Check sheet for the modelled part. Datum: model origin and axes. Units: mm. A direction names the side the tool comes from. Round coordinates to 2 decimals unless told otherwise and drop trailing zeros. Order: outer loops, then holes, each group sorted by start corner. A loop starts at its lowest first (then second) coordinate and runs counter-clockwise, first axis right, second up.
(1) Sectioned sample at A-A, the plane z = 15. Enter the section's corners in (x, y).
(2) Tool access check on faces 4 (the flat face through (0, -10, 28)), 5 (the flat face through (-15, 3, 0)), 6 (the flat face through (15, 3, 0)). Record the directions out of +Z, -Z, +X, -X, +Y, -Y that give a thin tool (end or side, any length) a straight path to the whole face; none if there is none.
(3) Depth check by flat-ended pin: pin 1 (4 mm diameter, centred on x = -6.5, z = -15, fed in from +Y); pin 2 (5 mm diameter, centred on x = 15, z = -8, fed in from -Y); pin 3 (6.5 mm diameter, centred on x = 15, z = 6, fed in from +Y). Enter the tip coordinate at first touch or a pass-through.
(4) Mould release check, pull along X, two halves, no side actions. Record for faces 1 (the flat face through (15, 0, 21)), 2 (the flat face through (-18.341, 0, 0)), 3 (the cylindrical face through (7.268, 2.289, -0.511)): released by +X, released by -X, zero draft, split by the parting line, or undercut.
(5) Sectioned sample at C-C, the plane x = 0. Enter the section's corners in (y, z), and give its area (3 significant figures).
(6) Sectioned sample at D-D, the plane z = 32.25. Enter the section's corners in (x, y), and give its area (3 significant figures).
(7) Sectioned sample at B-B, the plane y = 0. Enter the section's corners in (x, z), and give its area (3 significant figures).
(8) Thickness scan on probe 1 along Z at (x, y) = (10.05, 0); probe 2 along X at (y, z) = (0, 16); probe 3 along Y at (x, z) = (-4.5, 10.5). Record the ranges inside material, lowest first.
```python
from build123d import *

# Parameters (mm, degrees)
F0_R     = 12.7
F0_R_2   = 7.62
F1_DEPTH = 36.5
F3_DEPTH = 21
F4_W     = 43.0633045018
F4_H     = 8.1969123185
F4_H_2   = 6.7737210393
F5_DEPTH = 8.5
F8_D     = 3.3
F8_DEPTH = 30
F8_TIP   = 0.9914200214


with BuildPart() as f1:
    # F0 (on Top) → F1 (new body, symmetric)
    with BuildSketch(Plane.XY):
        Circle(F0_R)
        Circle(F0_R_2, mode=Mode.SUBTRACT)
    extrude(amount=F1_DEPTH, both=True)

    # F2 (on Top) → F3 (join, symmetric)
    with BuildSketch(Plane.XY):
        with BuildLine():
            Line((12.3405834546, -3), (18.3405834546, -3))
            Line((18.3405834546, -3), (18.3405834546, 3))
            Line((18.3405834546, 3), (12.3405834546, 3))
            ThreePointArc((12.3405834546, 3), (12.7, 0), (12.3405834546, -3))
        make_face()
        with BuildLine():
            Line((-12.3405834546, 3), (-18.3405834546, 3))
            Line((-18.3405834546, 3), (-18.3405834546, -3))
            Line((-18.3405834546, -3), (-12.3405834546, -3))
            ThreePointArc((-12.3405834546, -3), (-12.7, 0), (-12.3405834546, 3))
        make_face()
    extrude(amount=F3_DEPTH, both=True)

    # F4 (on face) → F5 (cut)
    with BuildSketch(Plane.XY.offset(36.5)):
        with Locations((0, -13.0984561592)):
            Rectangle(F4_W, F4_H)
        with Locations((0, 12.3868605196)):
            Rectangle(F4_W, F4_H_2)
    extrude(amount=-F5_DEPTH, mode=Mode.SUBTRACT)

    # F8
    with Locations(Plane.YZ.offset(12.7)):
        with Locations((0, 32.25)):
            Hole(F8_D / 2, depth=F8_DEPTH)
            with Locations((0, 0, -(F8_DEPTH + F8_TIP / 2))):  # 118° drill point
                Cone(0, F8_D / 2, F8_TIP, mode=Mode.SUBTRACT)


solid = f1.part
```
Derived:
1. outline: (-18.34, -3) - (-12.34, -3) arc R12.7 ccw to (12.34, -3) - (18.34, -3) - (18.34, 3) - (12.34, 3) arc R12.7 ccw to (-12.34, 3) - (-18.34, 3) - close; hole circle Ø15.24 at (0, 0)
2. face 4: +Z, +X, -X, -Y
2. face 5: +Z, -Z, -X, +Y
2. face 6: +Z, -Z, +X, +Y
3. pin 1: stops at y = 11.88
3. pin 2: stops at y = -3
3. pin 3: stops at y = 4.82
4. face 1: zero draft
4. face 2: released by -X
4. face 3: undercut
5. outline: (-12.7, -36.5) - (-7.62, -36.5) - (-7.62, 36.5) - (-9, 36.5) - (-9, 28) - (-12.7, 28) - close; (7.62, -36.5) - (12.7, -36.5) - (12.7, 28) - (9, 28) - (9, 36.5) - (7.62, 36.5) - close
5. area: 679 mm2
6. outline: (-12.59, -1.65) arc R12.7 ccw to (-8.96, -9) - (8.96, -9) arc R12.7 ccw to (12.59, -1.65) - (7.44, -1.65) arc R7.62 cw to (-7.44, -1.65) - close; (-12.59, 1.65) - (-7.44, 1.65) arc R7.62 cw to (7.44, 1.65) - (12.59, 1.65) arc R12.7 ccw to (8.96, 9) - (-8.96, 9) arc R12.7 ccw to start
6. area: 199 mm2
7. outline: (-18.34, -21) - (-12.7, -21) - (-12.7, -36.5) - (-7.62, -36.5) - (-7.62, 30.6) - (-12.7, 30.6) - (-12.7, 21) - (-18.34, 21) - close; (-12.7, 33.9) - (-7.62, 33.9) - (-7.62, 36.5) - (-12.7, 36.5) - close; (7.62, -36.5) - (12.7, -36.5) - (12.7, -21) - (18.34, -21) - (18.34, 21) - (12.7, 21) - (12.7, 30.6) - (7.62, 30.6) - close; (7.62, 33.9) - (12.7, 33.9) - (12.7, 36.5) - (7.62, 36.5) - close
7. area: 1,180 mm2
8. probe 1: z = -36.5 to 30.6, 33.9 to 36.5
8. probe 2: x = -18.34 to -7.62, 7.62 to 18.34
8. probe 3: y = -11.88 to -6.15, 6.15 to 11.88
